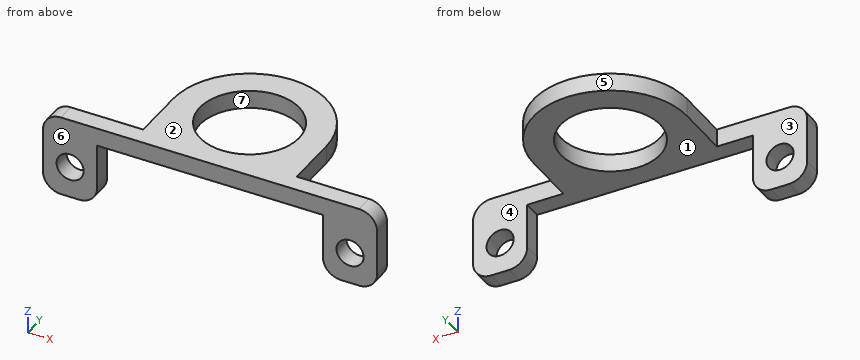
```python
from build123d import *

# Parameters (mm, degrees)
SKETCH_1_R      = 1.5
EXTRUDE_1_DEPTH = 2
SKETCH_2_R      = 5.5
EXTRUDE_2_DEPTH = 2
FILLET_1_R      = 2


with BuildPart() as part:
    # 草图1 → 凸台-拉伸1 (new body)
    with BuildSketch(Plane(origin=(0, 0, 0), x_dir=(1, 0, 0), z_dir=(0, 1, 0))):
        Polygon((-12.5, -3.5), (12.5, -3.5), (12.5, 3.5), (18.5, 3.5), (18.5, -3.5), (18.5, -5.5), (-18.5, -5.5), (-18.5, -3.5), (-18.5, 3.5), (-12.5, 3.5), align=None)
        with Locations(Location((-15.5, 0, 0), (0, 0, 270))):
            Circle(SKETCH_1_R, mode=Mode.SUBTRACT)
        with Locations(Location((15.5, 0, 0), (0, 0, 90))):
            Circle(SKETCH_1_R, mode=Mode.SUBTRACT)
    extrude(amount=EXTRUDE_1_DEPTH)

    # 草图2 → 凸台-拉伸2 (add)
    with BuildSketch(Plane.XY.offset(5.5)):
        with BuildLine():
            Line((-8.5, 8), (-8.5, 0))
            Line((-8.5, 0), (8.5, 0))
            Line((8.5, 0), (8.5, 8))
            ThreePointArc((8.5, 8), (0, 16.5), (-8.5, 8))
        make_face()
        with Locations((0, 8)):
            Circle(SKETCH_2_R, mode=Mode.SUBTRACT)
    extrude(amount=-EXTRUDE_2_DEPTH)

    # 圆角1
    fillet_1_edges = [part.edges().sort_by_distance(p)[0] for p in [
        (12.5, 1, -3.5),
        (18.5, 1, -3.5),
        (18.5, 1, 5.5),
        (-18.5, 1, 5.5),
        (-18.5, 1, -3.5),
        (-12.5, 1, -3.5),
    ]]
    fillet(fillet_1_edges, radius=FILLET_1_R)


solid = part.part
```
For this review, take the finished solid that the model builds, in its own axes (mm). Face numbers are marked on the shaded views. A direction names the side the tool comes from. Give positions to 0.01 mm unless a question says otherwise; leave off trailing zeros. Write each loop counter-clockwise with the first axis right and the second up, starting at its lowest first coordinate (ties: lowest second). Pieces come first, ordered by that corner, then holes.
Item 1: Take a section at C-C (y = 11). Give the boundary of the cut face in (x, z), and give its area (3 significant figures).
Item 2: Wall thickness on probe 1 along X at (y, z) = (1.4, 0); probe 2 along Y at (x, z) = (0, 4.95); probe 3 along Z at (x, y) = (-11.5, 0.75): over which ranges is each line inside the solid? List them lowest first.
Item 3: Machinability: for the marked faces 1, 2, 3 and 4, which of the approach directions +Z, -Z, +X, -X, +Y, -Y give a long, thin tool a straight path to every point of the face, cutting with its end or side? Answer none if there is none.
Item 4: Take a section at D-D (z = 4.75). Give the boundary of the cut face in (x, y), and give its area (3 significant figures).
Item 5: Take a section at A-A (z = 0). Give the boundary of the cut face in (x, y).
Item 6: Insertion check: P1, Ø8, axis at x = -7.5, y = 11.5, coming from the -Z side; P2, Ø1, axis at y = 6, z = 4.5, coming from the +X side; P3, Ø5, axis at x = 14.5, z = 1.5, coming from the +Y side; P4, Ø6, axis at x = -2.5, y = 3.5, coming from the +Z side. Each pin has a flat end and moves straight along its axis. Give the tip position at first contact, or say it passes through.
Item 7: The part is to be moulded in two halves that separate along X. For the marked faces 5, 6 and 7, say which applies: +X half, -X half, draft (parallel to the pull), parting line (faces both ways), or undercut.
Item 8: Take a section at B-B (x = 0). Give the boundary of the cut face in (y, z), and give its area (3 significant figures).
Established:
1. outline: (-7.95, 3.5) - (-4.61, 3.5) - (-4.61, 5.5) - (-7.95, 5.5) - close; (4.61, 3.5) - (7.95, 3.5) - (7.95, 5.5) - (4.61, 5.5) - close
1. area: 13.4 mm2
2. probe 1: x = -18.5 to -17, -14 to -12.5, 12.5 to 14, 17 to 18.5
2. probe 2: y = 0 to 2.5, 13.5 to 16.5
2. probe 3: z = 3.5 to 5.5
3. face 1: -Z, +Y, -Y
3. face 2: +Z, +X, -X, +Y, -Y
3. face 3: +Z, -Z, -X, +Y
3. face 4: +Z, -Z, +X, +Y
4. outline: (-18.06, 0) - (18.06, 0) - (18.06, 2) - (8.5, 2) - (8.5, 8) arc R8.5 ccw to (-8.5, 8) - (-8.5, 2) - (-18.06, 2) - close; hole circle Ø11 at (0, 8)
4. area: 193 mm2
5. outline: (-18.5, 0) - (-17, 0) - (-17, 2) - (-18.5, 2) - close; (-14, 0) - (-12.5, 0) - (-12.5, 2) - (-14, 2) - close; (12.5, 0) - (14, 0) - (14, 2) - (12.5, 2) - close; (17, 0) - (18.5, 0) - (18.5, 2) - (17, 2) - close
6. P1: stops at z = 3.5
6. P2: stops at x = 8.5
6. P3: stops at y = 2
6. P4: stops at z = 5.5
7. face 5: parting line
7. face 6: draft
7. face 7: undercut
8. outline: (0, 3.5) - (2.5, 3.5) - (2.5, 5.5) - (0, 5.5) - close; (13.5, 3.5) - (16.5, 3.5) - (16.5, 5.5) - (13.5, 5.5) - close
8. area: 11.0 mm2
